```python
from build123d import *

# Parameters (mm, degrees)
SKETCH1_W                    = 15
SKETCH1_H                    = 45.15
BASE_FLANGE1_DEPTH           = 3.175
EDGE_FLANGE1_STRIP_W         = 14.7
EDGE_FLANGE1_STRIP_H         = 3.175
EDGE_FLANGE1_STRIP_CUT_DEPTH = 15
EDGE_FLANGE1_DEPTH           = 15
EDGE_FLANGE2_STRIP_W         = 14.7
EDGE_FLANGE2_STRIP_H         = 3.175
EDGE_FLANGE2_STRIP_CUT_DEPTH = 15
EDGE_FLANGE2_DEPTH           = 15
M5_CLEARANCE_HOLE2_D         = 5.5
M5_CLEARANCE_HOLE1_D         = 5.5
M3_CLEARANCE_HOLE1_D         = 3.4
FILLET1_R                    = 3.175


# Sheet-metal steps are written as plain solids
with BuildPart() as part:
    # Sketch1 → Base-Flange1 (new body)
    with BuildSketch(Plane(origin=(0, 0, 0), x_dir=(1, 0, 0), z_dir=(0, 1, 0))):
        Rectangle(SKETCH1_W, SKETCH1_H)
    extrude(amount=-BASE_FLANGE1_DEPTH)

    # Edge-Flange1 strip (across the edge) → Edge-Flange1 strip cut (cut)
    with BuildSketch(Plane(origin=(7.5, 0, -22.575), x_dir=(0, 0, 1), z_dir=(-1, 0, 0))):
        with Locations((-3.175, -1.5875)):
            Rectangle(EDGE_FLANGE1_STRIP_W, EDGE_FLANGE1_STRIP_H)
    extrude(amount=EDGE_FLANGE1_STRIP_CUT_DEPTH, mode=Mode.SUBTRACT)

    # Edge-Flange1 section (across the edge) → Edge-Flange1 (add)
    with BuildSketch(Plane(origin=(7.5, 0, -22.575), x_dir=(0, 0, 1), z_dir=(-1, 0, 0))):
        with BuildLine():
            Line((0, 1), (0, 45.825))
            Line((0, 45.825), (3.175, 45.825))
            Line((3.175, 45.825), (3.175, 1))
            ThreePointArc((3.175, 1), (3.467893219, 0.292893219), (4.175, 0))
            Line((4.175, 0), (4.175, -3.175))
            ThreePointArc((4.175, -3.175), (1.222829189, -1.952170811), (0, 1))
        make_face()
    extrude(amount=EDGE_FLANGE1_DEPTH)

    # Edge-Flange2 strip (across the edge) → Edge-Flange2 strip cut (cut)
    with BuildSketch(Plane(origin=(-7.5, 45.825, -22.575), x_dir=(0, -1, 0), z_dir=(1, 0, 0))):
        with Locations((-3.175, -1.5875)):
            Rectangle(EDGE_FLANGE2_STRIP_W, EDGE_FLANGE2_STRIP_H)
    extrude(amount=EDGE_FLANGE2_STRIP_CUT_DEPTH, mode=Mode.SUBTRACT)

    # Edge-Flange2 section (across the edge) → Edge-Flange2 (add)
    with BuildSketch(Plane(origin=(-7.5, 45.825, -22.575), x_dir=(0, -1, 0), z_dir=(1, 0, 0))):
        with BuildLine():
            Line((0, 1), (0, 53.825))
            Line((0, 53.825), (3.175, 53.825))
            Line((3.175, 53.825), (3.175, 1))
            ThreePointArc((3.175, 1), (3.467893219, 0.292893219), (4.175, 0))
            Line((4.175, 0), (4.175, -3.175))
            ThreePointArc((4.175, -3.175), (1.222829189, -1.952170811), (0, 1))
        make_face()
    extrude(amount=EDGE_FLANGE2_DEPTH)

    # M5 Clearance Hole2 (through all)
    with Locations(Plane(origin=(0, 0, 0), x_dir=(1, 0, 0), z_dir=(0, 1, 0))):
        with Locations((0, -16.575)):
            Hole(M5_CLEARANCE_HOLE2_D / 2)

    # M5 Clearance Hole1 (through all)
    with Locations(Plane(origin=(0, 45.825, 0), x_dir=(1, 0, 0), z_dir=(0, 1, 0))):
        with Locations((0, 70.4)):
            Hole(M5_CLEARANCE_HOLE1_D / 2)

    # M3 Clearance Hole1 (through all)
    with Locations(Plane(origin=(0, 45.825, 0), x_dir=(1, 0, 0), z_dir=(0, 1, 0))):
        with Locations((0, 28.9)):
            Hole(M3_CLEARANCE_HOLE1_D / 2)

    # Fillet1
    fillet1_edges = [part.edges().sort_by_distance(p)[0] for p in [
        (-7.5, 44.2375, -76.4),
        (7.5, 44.2375, -76.4),
        (7.5, -1.5875, 22.575),
        (-7.5, -1.5875, 22.575),
    ]]
    fillet(fillet1_edges, radius=FILLET1_R)


solid = part.part
```
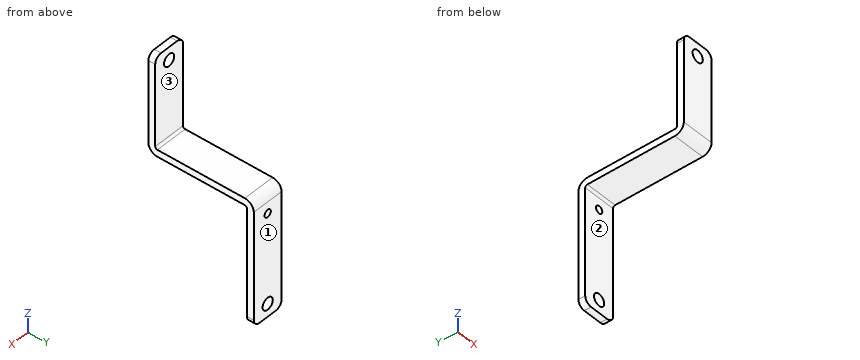
Part model, mm, in its own coordinate system. Face numbers are marked on the shaded views. A direction names the side the tool comes from. Coordinates: 2 decimals unless noted, no trailing zeros. Write each loop counter-clockwise with the first axis right and the second up, starting at its lowest first coordinate (ties: lowest second). Pieces come first, ordered by that corner, then holes.
Item 1: Slice it at B-B (x = 0). Write the cut outline in (y, z) (3 decimals), and give its area (3 significant figures).
Item 2: Slice it at C-C (z = -70.4). Write the cut outline in (x, y) (3 decimals).
Item 3: Pin check, flat tips, straight feed: pin 1 (7.5 mm diameter, centred on x = -3.5, y = 28.5, fed in from -Z) (3 decimals); pin 2 (7 mm diameter, centred on x = 0, z = -70.4, fed in from -Y); pin 3 (2 mm diameter, centred on x = 0, z = -28.9, fed in from -Y); pin 4 (9 mm diameter, centred on x = 0, z = 16.575, fed in from +Y). Stop position of each tip, or through.
Item 4: Slice it at D-D (x = -5.25). Write the cut outline in (y, z) (3 decimals).
Item 5: Probe line 1 (Z direction, x = 0, y = 44.1); line 2 (X direction, y = 44.95, z = -28.9); line 3 (Z direction, x = 0, y = 44.3). List the from-to ranges inside material, lowest first.
Item 6: Which spindle directions (+Z, -Z, +X, -X, +Y, -Y) get a long thin tool onto all of the face, cutting with end or side? Do the marked faces 1, 2 and 3. Say none if no direction does.
Item 7: Slice it at A-A (z = -28.9). Write the cut outline in (x, y) (3 decimals).
Results found:
1. outline: (-3.175, -18.4) arc R4.175 ccw to (1, -22.575) - (41.65, -22.575) arc R1 cw to (42.65, -23.575) - (42.65, -27.2) - (45.825, -27.2) - (45.825, -23.575) arc R4.175 ccw to (41.65, -19.4) - (1, -19.4) arc R1 cw to (0, -18.4) - (0, 13.825) - (-3.175, 13.825) - close; (-3.175, 19.325) - (0, 19.325) - (0, 22.575) - (-3.175, 22.575) - close; (42.65, -76.4) - (45.825, -76.4) - (45.825, -73.15) - (42.65, -73.15) - close; (42.65, -67.65) - (45.825, -67.65) - (45.825, -30.6) - (42.65, -30.6) - close
1. area: 407 mm2
2. outline: (-7.5, 42.65) - (-2.75, 42.65) - (-2.75, 45.825) - (-7.5, 45.825) - close; (2.75, 42.65) - (7.5, 42.65) - (7.5, 45.825) - (2.75, 45.825) - close
3. pin 1: stops at z = -22.575
3. pin 2: stops at y = 42.65
3. pin 3: passes through
3. pin 4: stops at y = 0
4. outline: (-3.175, -18.4) arc R4.175 ccw to (1, -22.575) - (41.65, -22.575) arc R1 cw to (42.65, -23.575) - (42.65, -76.262) - (45.825, -76.262) - (45.825, -23.575) arc R4.175 ccw to (41.65, -19.4) - (1, -19.4) arc R1 cw to (0, -18.4) - (0, 22.437) - (-3.175, 22.437) - close
5. line 1: z = -76.4 to -73.15, -67.65 to -30.6, -27.2 to -20.19
5. line 2: x = -7.5 to -1.7, 1.7 to 7.5
5. line 3: z = -76.4 to -73.15, -67.65 to -30.6, -27.2 to -20.35
6. face 1: +Z, -Z, +X, -X, +Y
6. face 2: -Z, +X, -X, -Y
6. face 3: +Z, +X, -X, +Y
7. outline: (-7.5, 42.65) - (-1.7, 42.65) - (-1.7, 45.825) - (-7.5, 45.825) - close; (1.7, 42.65) - (7.5, 42.65) - (7.5, 45.825) - (1.7, 45.825) - close
